from build123d import *

# Parameters (mm, degrees)
MODEL_R         = 3
MODEL_R_2       = 2.35
MODEL_R_3       = 5
MODEL_W         = 2.2
MODEL_H         = 10
EXTRUDE_1_DEPTH = 2


with BuildPart() as part:
    # Model → 凸台-拉伸1 (new body)
    with BuildSketch(Plane.XY):
        with BuildLine():
            Line((42.207834759, 34.585721775), (42.207834759, 37.585721775))
            Line((42.207834759, 37.585721775), (4.478222617, 37.585721775))
            Line((4.478222617, 37.585721775), (4.478222617, 34.585721775))
            Line((4.478222617, 34.585721775), (13.878222617, 34.585721775))
            Line((13.878222617, 34.585721775), (13.878222617, 5.585721775))
            Line((13.878222617, 5.585721775), (4.478222617, 5.585721775))
            Line((4.478222617, 5.585721775), (4.478222617, 2.585721775))
            Line((4.478222617, 2.585721775), (42.207834759, 2.585721775))
            Line((42.207834759, 2.585721775), (42.207834759, 5.585721775))
            ThreePointArc((42.207834759, 5.585721775), (46.241179833, 9.551811246), (50.207269305, 5.518466173))
            Line((50.207269305, 5.518466173), (50.205774509, 2.585721775))
            Line((50.205774509, 2.585721775), (62.206804634, 2.585721775))
            Line((62.206804634, 2.585721775), (62.206804634, 10.085721775))
            ThreePointArc((62.206804634, 10.085721775), (62.646144463, 11.146381946), (63.706804634, 11.585721775))
            Line((63.706804634, 11.585721775), (83.706804634, 11.585721775))
            ThreePointArc((83.706804634, 11.585721775), (84.767464806, 11.146381946), (85.206804634, 10.085721775))
            Line((85.206804634, 10.085721775), (85.206804634, 2.585721775))
            Line((85.206804634, 2.585721775), (91.206804634, 2.585721775))
            Line((91.206804634, 2.585721775), (91.206804634, 10.085721775))
            ThreePointArc((91.206804634, 10.085721775), (91.646144463, 11.146381946), (92.706804634, 11.585721775))
            Line((92.706804634, 11.585721775), (115.049506416, 11.585721775))
            ThreePointArc((115.049506416, 11.585721775), (115.921363706, 11.306321981), (116.468425335, 10.572208261))
            Line((116.468425335, 10.572208261), (119.206649273, 2.585721775))
            Line((119.206649273, 2.585721775), (123.706021861, 2.585721775))
            Line((123.706021861, 2.585721775), (123.706021861, 6.085721775))
            ThreePointArc((123.706021861, 6.085721775), (124.145361689, 7.146381946), (125.206021861, 7.585721775))
            Line((125.206021861, 7.585721775), (159.806021861, 7.585721775))
            ThreePointArc((159.806021861, 7.585721775), (160.866682033, 7.146381946), (161.306021861, 6.085721775))
            Line((161.306021861, 6.085721775), (161.306021861, 2.585721775))
            Line((161.306021861, 2.585721775), (176.857875106, 2.585721775))
            ThreePointArc((176.857875106, 2.585721775), (182.857875106, 8.585721775), (176.857875106, 14.585721775))
            Line((176.857875106, 14.585721775), (172.375964349, 14.585721775))
            Line((172.375964349, 14.585721775), (172.375964349, 25.585721775))
            Line((172.375964349, 25.585721775), (176.857875106, 25.585721775))
            ThreePointArc((176.857875106, 25.585721775), (182.857875106, 31.585721775), (176.857875106, 37.585721775))
            Line((176.857875106, 37.585721775), (161.306021861, 37.585721775))
            Line((161.306021861, 37.585721775), (161.306021861, 34.085721775))
            ThreePointArc((161.306021861, 34.085721775), (160.866682033, 33.025061603), (159.806021861, 32.585721775))
            Line((159.806021861, 32.585721775), (125.206021861, 32.585721775))
            ThreePointArc((125.206021861, 32.585721775), (124.145361689, 33.025061603), (123.706021861, 34.085721775))
            Line((123.706021861, 34.085721775), (123.706021861, 37.585721775))
            Line((123.706021861, 37.585721775), (119.206649273, 37.585721775))
            Line((119.206649273, 37.585721775), (116.468425335, 29.599235288))
            ThreePointArc((116.468425335, 29.599235288), (115.921363706, 28.865121568), (115.049506416, 28.585721775))
            Line((115.049506416, 28.585721775), (92.706804634, 28.585721775))
            ThreePointArc((92.706804634, 28.585721775), (91.646144463, 29.025061603), (91.206804634, 30.085721775))
            Line((91.206804634, 30.085721775), (91.206804634, 37.585721775))
            Line((91.206804634, 37.585721775), (85.206804634, 37.585721775))
            Line((85.206804634, 37.585721775), (85.206804634, 30.085721775))
            ThreePointArc((85.206804634, 30.085721775), (84.767464806, 29.025061603), (83.706804634, 28.585721775))
            Line((83.706804634, 28.585721775), (63.706804634, 28.585721775))
            ThreePointArc((63.706804634, 28.585721775), (62.646144463, 29.025061603), (62.206804634, 30.085721775))
            Line((62.206804634, 30.085721775), (62.206804634, 37.585721775))
            Line((62.206804634, 37.585721775), (50.205774509, 37.585721775))
            Line((50.205774509, 37.585721775), (50.205774509, 34.585721775))
            ThreePointArc((50.205774509, 34.585721775), (46.206804634, 30.501548086), (42.207834759, 34.585721775))
        make_face()
        with Locations((176.745324773, 8.585721775)):
            Circle(MODEL_R, mode=Mode.SUBTRACT)
        with Locations((176.745324773, 31.585721775)):
            Circle(MODEL_R, mode=Mode.SUBTRACT)
        with Locations((116.856649273, 20.085721775)):
            Circle(MODEL_R_2, mode=Mode.SUBTRACT)
        with Locations((46.479868031, 20.085721775)):
            Circle(MODEL_R_3, mode=Mode.SUBTRACT)
        with BuildLine():
            Line((161.306021861, 22.585721775), (161.306021861, 29.085721775))
            ThreePointArc((161.306021861, 29.085721775), (160.866682033, 30.146381946), (159.806021861, 30.585721775))
            Line((159.806021861, 30.585721775), (125.206021861, 30.585721775))
            ThreePointArc((125.206021861, 30.585721775), (124.145361689, 30.146381946), (123.706021861, 29.085721775))
            Line((123.706021861, 29.085721775), (123.706021861, 22.585721775))
            ThreePointArc((123.706021861, 22.585721775), (124.145361689, 21.525061603), (125.206021861, 21.085721775))
            Line((125.206021861, 21.085721775), (159.806021861, 21.085721775))
            ThreePointArc((159.806021861, 21.085721775), (160.866682033, 21.525061603), (161.306021861, 22.585721775))
        make_face(mode=Mode.SUBTRACT)
        with BuildLine():
            Line((123.706021861, 17.585721775), (123.706021861, 11.085721775))
            ThreePointArc((123.706021861, 11.085721775), (124.145361689, 10.025061603), (125.206021861, 9.585721775))
            Line((125.206021861, 9.585721775), (159.806021861, 9.585721775))
            ThreePointArc((159.806021861, 9.585721775), (160.866682033, 10.025061603), (161.306021861, 11.085721775))
            Line((161.306021861, 11.085721775), (161.306021861, 17.585721775))
            ThreePointArc((161.306021861, 17.585721775), (160.866682033, 18.646381946), (159.806021861, 19.085721775))
            Line((159.806021861, 19.085721775), (125.206021861, 19.085721775))
            ThreePointArc((125.206021861, 19.085721775), (124.145361689, 18.646381946), (123.706021861, 17.585721775))
        make_face(mode=Mode.SUBTRACT)
        with Locations((56.506804634, 12.585721775)):
            Rectangle(MODEL_W, MODEL_H, mode=Mode.SUBTRACT)
        with Locations((56.506804634, 27.585721775)):
            Rectangle(MODEL_W, MODEL_H, mode=Mode.SUBTRACT)
        with Locations((165.406021861, 12.585721775)):
            Rectangle(MODEL_W, MODEL_H, mode=Mode.SUBTRACT)
        with Locations((165.406021861, 27.585721775)):
            Rectangle(MODEL_W, MODEL_H, mode=Mode.SUBTRACT)
        with Locations((120.306649273, 12.585721775)):
            Rectangle(MODEL_W, MODEL_H, mode=Mode.SUBTRACT)
        with Locations((120.306649273, 27.585721775)):
            Rectangle(MODEL_W, MODEL_H, mode=Mode.SUBTRACT)
        Polygon((87.206804634, 7.585721775), (89.406804634, 7.585721775), (89.406791039, 17.583389823), (87.206804634, 17.585721775), align=None, mode=Mode.SUBTRACT)
        Polygon((87.253377966, 32.591005683), (89.453377966, 32.591005683), (89.406734823, 22.591005683), (87.253377966, 22.591005683), align=None, mode=Mode.SUBTRACT)
        with BuildLine():
            Line((62.706804634, 13.585721775), (83.706804634, 13.585721775))
            ThreePointArc((83.706804634, 13.585721775), (84.767464806, 14.025061603), (85.206804634, 15.085721775))
            Line((85.206804634, 15.085721775), (85.206804634, 25.085721775))
            ThreePointArc((85.206804634, 25.085721775), (84.767464806, 26.146381946), (83.706804634, 26.585721775))
            Line((83.706804634, 26.585721775), (62.706804634, 26.585721775))
            ThreePointArc((62.706804634, 26.585721775), (61.646144463, 26.146381946), (61.206804634, 25.085721775))
            Line((61.206804634, 25.085721775), (61.206804634, 15.085721775))
            ThreePointArc((61.206804634, 15.085721775), (61.646144463, 14.025061603), (62.706804634, 13.585721775))
        make_face(mode=Mode.SUBTRACT)
        with BuildLine():
            Line((113.335220701, 26.585721775), (92.706804634, 26.585721775))
            ThreePointArc((92.706804634, 26.585721775), (91.646144463, 26.146381946), (91.206804634, 25.085721775))
            Line((91.206804634, 25.085721775), (91.206804634, 15.085721775))
            ThreePointArc((91.206804634, 15.085721775), (91.646144463, 14.025061603), (92.706804634, 13.585721775))
            Line((92.706804634, 13.585721775), (113.335220701, 13.585721775))
            ThreePointArc((113.335220701, 13.585721775), (114.555820908, 14.213864484), (114.75413962, 15.572208261))
            Line((114.75413962, 15.572208261), (113.37344464, 19.599235288))
            ThreePointArc((113.37344464, 19.599235288), (113.292363558, 20.085721775), (113.37344464, 20.572208261))
            Line((113.37344464, 20.572208261), (114.75413962, 24.599235288))
            ThreePointArc((114.75413962, 24.599235288), (114.555820908, 25.957579065), (113.335220701, 26.585721775))
        make_face(mode=Mode.SUBTRACT)
        with BuildLine():
            Line((18.477950078, 22.799320708), (37.681937895, 22.799320708))
            ThreePointArc((37.681937895, 22.799320708), (38.742598067, 23.238660536), (39.181937895, 24.299320708))
            Line((39.181937895, 24.299320708), (39.181937895, 30.799320708))
            ThreePointArc((39.181937895, 30.799320708), (38.742598067, 31.859980879), (37.681937895, 32.299320708))
            Line((37.681937895, 32.299320708), (18.477950078, 32.299320708))
            ThreePointArc((18.477950078, 32.299320708), (17.417289906, 31.859980879), (16.977950078, 30.799320708))
            Line((16.977950078, 30.799320708), (16.977950078, 24.299320708))
            ThreePointArc((16.977950078, 24.299320708), (17.417289906, 23.238660536), (18.477950078, 22.799320708))
        make_face(mode=Mode.SUBTRACT)
        with BuildLine():
            Line((18.477950078, 17.372122842), (37.681937895, 17.372122842))
            ThreePointArc((37.681937895, 17.372122842), (38.742598067, 16.932783014), (39.181937895, 15.872122842))
            Line((39.181937895, 15.872122842), (39.181937895, 9.372122842))
            ThreePointArc((39.181937895, 9.372122842), (38.742598067, 8.31146267), (37.681937895, 7.872122842))
            Line((37.681937895, 7.872122842), (18.477950078, 7.872122842))
            ThreePointArc((18.477950078, 7.872122842), (17.417289906, 8.31146267), (16.977950078, 9.372122842))
            Line((16.977950078, 9.372122842), (16.977950078, 15.872122842))
            ThreePointArc((16.977950078, 15.872122842), (17.417289906, 16.932783014), (18.477950078, 17.372122842))
        make_face(mode=Mode.SUBTRACT)
    extrude(amount=EXTRUDE_1_DEPTH)


solid = part.part
Verification items for the finished model (mm, model axes). A direction names the side the tool comes from. Round coordinates to 2 decimals unless told otherwise and drop trailing zeros. Loops run counter-clockwise (first coordinate to the right, second up) from the corner with the lowest first, then second, coordinate; pieces in that order, holes last. Notation, with made-up numbers: (87.25, 74.5) - (141.25, 74.5) arc R18 cw to (141.25, 93.5) - close; hole circle Ø6 at (81.25, 17.5). An arc over 180 degrees is marked (long way). Answer in a Markdown table with one row per item. Add a question column.
Q1. Release check for a two-part mould opening along X. For faces 1 (the face through (182.856, 8.454, 0.986)), 2 (the face through (115.12, 21.67, 0.99)), 3 (the face through (46.15, 9.55, 0.99)), 4 (the face through (92, 28, 0)) record: pulls with the +X half, pulls with the -X half, needs draft (parallel to the pull), parting line crosses it, or undercut.
Q2. Gauge pin test, flat ends, axial feed: pin 1 (1 mm diameter, centred on x = 145, z = 1, fed in from -Y); pin 2 (1 mm diameter, centred on y = 30, z = 1.5, fed in from -X). Record the tip position at first contact, or that the pin passes through.
Q3. Section check A-A on x = 72. Enter the section's corners in (y, z), plus the area to 3 significant figures.
Q4. Material ranges on line 1 (X direction, y = 20.5, z = 0.7); line 2 (Y direction, x = 55.5, z = 1.65); line 3 (Y direction, x = 139.5, z = 0.65), recorded low to high.
Q5. Tool access check on faces 5 (the face through (117.857, 33.648, 0.986)), 6 (the face through (179.607, 9.487, 0.986)), 7 (the face through (117.82, 6.63, 0.99)). Record the directions out of +Z, -Z, +X, -X, +Y, -Y that give a thin tool (end or side, any length) a straight path to the whole face; none if there is none.
Q6. Section check B-B on x = 127. Enter the section's corners in (y, z), plus the area to 3 significant figures.
Q7. Section check C-C on z = 0.4. State how many separate pieces and enclosed holes the cut face has, plus the area to 3 significant figures.
Found:
| question | item | result |
|---|---|---|
| 1 | face 1 | pulls with the +X half |
| 1 | face 2 | undercut |
| 1 | face 3 | undercut |
| 1 | face 4 | needs draft |
| 2 | pin 1 | stops at y = 7.59 |
| 2 | pin 2 | stops at x = 13.88 |
| 3 | outline | (11.59, 0) - (13.59, 0) - (13.59, 2) - (11.59, 2) - close; (26.59, 0) - (28.59, 0) - (28.59, 2) - (26.59, 2) - close |
| 3 | area | 8.00 mm² |
| 4 | line 1 | x = 13.88 to 41.5, 51.46 to 61.21, 85.21 to 91.21, 113.35 to 114.54, 119.17 to 172.38 |
| 4 | line 2 | y = 2.59 to 7.59, 17.59 to 22.59, 32.59 to 37.59 |
| 4 | line 3 | y = 7.59 to 9.59, 19.09 to 21.09, 30.59 to 32.59 |
| 5 | face 5 | +Z, -Z, +Y |
| 5 | face 6 | +Z, -Z |
| 5 | face 7 | +Z, -Z, -Y |
| 6 | outline | (7.59, 0) - (9.59, 0) - (9.59, 2) - (7.59, 2) - close; (19.09, 0) - (21.09, 0) - (21.09, 2) - (19.09, 2) - close; (30.59, 0) - (32.59, 0) - (32.59, 2) - (30.59, 2) - close |
| 6 | area | 12.0 mm² |
| 7 | separate pieces | 1 |
| 7 | enclosed holes | 18 |
| 7 | area | 2,400 mm² |
